from build123d import *

# Parameters (mm, degrees)
SKETCH_1_W               = 164.2
SKETCH_1_H               = 104.2
EXTRUDE_1_DEPTH          = 8
SKETCH_2_R               = 0.3
CUT_EXTRUDE_1_DEPTH      = 98.564440243
CUT_EXTRUDE_2_DEPTH      = 5.9
SKETCH_5_W               = 148.4
SKETCH_5_H               = 100.2
CUT_EXTRUDE_5_DEPTH      = 1.2
SKETCH_6_W               = 164.2
SKETCH_6_H               = 104.2
SKETCH_6_W_2             = 148.4
SKETCH_6_H_2             = 100.2
EXTRUDE_2_DEPTH          = 3
CUT_EXTRUDE_6_DEPTH      = 132.336400133
CUT_EXTRUDE_6_DEPTH_BACK = 132.336400133
SKETCH_7_R               = 0.75
CUT_EXTRUDE_START        = -2
SKETCH_7_3_R             = 1
SKETCH_7_3_R_2           = 0.75
CUT_EXTRUDE_7_DEPTH      = 1
CUT_EXTRUDE_START_2      = 101.2
SKETCH_7_4_R             = 1
SKETCH_7_4_R_2           = 0.75
CUT_EXTRUDE_8_DEPTH      = 1
SKETCH_8_R               = 0.75
CUT_EXTRUDE_9_DEPTH      = 171.644953046
CUT_EXTRUDE_START_3      = -0.9
SKETCH_8_3_R             = 1
SKETCH_8_3_R_2           = 0.75
CUT_EXTRUDE_10_DEPTH     = 1
SKETCH_3_W               = 145.9
SKETCH_3_H               = 96.2
SKETCH_3_W_2             = 10.3
SKETCH_3_H_2             = 30.95
CUT_EXTRUDE_11_DEPTH     = 4.8
SKETCH_9_W               = 164.2
SKETCH_9_H               = 104.2
CUT_EXTRUDE_12_DEPTH     = 2.4


with BuildPart() as part:
    # 草图1 → 凸台-拉伸1 (new body)
    with BuildSketch(Plane(origin=(0, 0, 0), x_dir=(1, 0, 0), z_dir=(0, 1, 0))):
        Rectangle(SKETCH_1_W, SKETCH_1_H)
    extrude(amount=EXTRUDE_1_DEPTH)

    # 草图2 → 切除-拉伸1 (cut, through all)
    with BuildSketch(Plane(origin=(0, 8, 0), x_dir=(1, 0, 0), z_dir=(0, 1, 0))):
        with Locations(Location((-74, 11.5, 0), (0, 0, 270))):
            Circle(SKETCH_2_R)
        with Locations(Location((-74, -11.5, 0), (0, 0, 270))):
            Circle(SKETCH_2_R)
        with BuildLine():
            Line((-76.2, -8.05), (-76.2, 8.05))
            ThreePointArc((-76.2, 8.05), (-74, 10.25), (-71.8, 8.05))
            Line((-71.8, 8.05), (-71.8, -8.05))
            ThreePointArc((-71.8, -8.05), (-74, -10.25), (-76.2, -8.05))
        make_face()
    extrude(amount=-CUT_EXTRUDE_1_DEPTH, mode=Mode.SUBTRACT)

    # 草图2<3> → 切除-拉伸2 (cut)
    with BuildSketch(Plane(origin=(0, 8, 0), x_dir=(1, 0, 0), z_dir=(0, 1, 0))):
        with BuildLine():
            Line((-71.8, 10.95), (-71.8, -10.95))
            ThreePointArc((-71.8, -10.95), (-74, -13.15), (-76.2, -10.95))
            Line((-76.2, -10.95), (-76.2, 10.95))
            ThreePointArc((-76.2, 10.95), (-74, 13.15), (-71.8, 10.95))
        make_face()
    extrude(amount=-CUT_EXTRUDE_2_DEPTH, mode=Mode.SUBTRACT)

    # 草图5 → 切除-拉伸5 (cut)
    with BuildSketch(Plane.XZ):
        with Locations((6, 0)):
            Rectangle(SKETCH_5_W, SKETCH_5_H)
    extrude(amount=-CUT_EXTRUDE_5_DEPTH, mode=Mode.SUBTRACT)

    # 草图6 → 凸台-拉伸2 (add)
    with BuildSketch(Plane.XZ):
        Rectangle(SKETCH_6_W, SKETCH_6_H)
        with BuildLine():
            ThreePointArc((-71.8, -10.95), (-74.1, -13.25), (-76.4, -10.95))
            Line((-76.4, -10.95), (-76.4, -5.229910312))
            ThreePointArc((-76.4, -5.229910312), (-77.793738469, -4.481131324), (-78.35, -3))
            Line((-78.35, -3), (-78.35, 3))
            ThreePointArc((-78.35, 3), (-77.793738469, 4.481131324), (-76.4, 5.229910312))
            Line((-76.4, 5.229910312), (-76.4, 10.95))
            ThreePointArc((-76.4, 10.95), (-74.1, 13.25), (-71.8, 10.95))
            Line((-71.8, 10.95), (-71.8, 8.05))
            Line((-71.8, 8.05), (-71.8, 2.229910312))
            ThreePointArc((-71.8, 2.229910312), (-70.406261531, 1.481131324), (-69.85, 0))
            ThreePointArc((-69.85, 0), (-70.406261531, -1.481131324), (-71.8, -2.229910312))
            Line((-71.8, -2.229910312), (-71.8, -8.05))
            Line((-71.8, -8.05), (-71.8, -10.95))
        make_face(mode=Mode.SUBTRACT)
        with Locations((6, 0)):
            Rectangle(SKETCH_6_W_2, SKETCH_6_H_2, mode=Mode.SUBTRACT)
    extrude(amount=EXTRUDE_2_DEPTH)

    # 草图7 → 切除-拉伸6 (cut, two sides: drawn at the far end of the back side and taken through both)
    with BuildSketch(Plane.XY.offset(-50.1).offset(-CUT_EXTRUDE_6_DEPTH_BACK)):
        with Locations((6, -1)):
            Circle(SKETCH_7_R)
        with Locations((-54, -1)):
            Circle(SKETCH_7_R)
        with Locations((66, -1)):
            Circle(SKETCH_7_R)
    extrude(amount=CUT_EXTRUDE_6_DEPTH + CUT_EXTRUDE_6_DEPTH_BACK, mode=Mode.SUBTRACT)

    # 草图7<3> → 切除-拉伸7 (cut)
    # profile 1 of 3: a face of its own
    with BuildSketch(Plane.XY.offset(-50.1).offset(CUT_EXTRUDE_START)):
        with Locations((6, -1)):
            Circle(SKETCH_7_3_R)
        with Locations((6, -1)):
            Circle(SKETCH_7_3_R_2, mode=Mode.SUBTRACT)
    # profile 2 of 3: a face of its own
    with BuildSketch(Plane.XY.offset(-50.1).offset(CUT_EXTRUDE_START)):
        with Locations((66, -1)):
            Circle(SKETCH_7_3_R)
        with Locations((66, -1)):
            Circle(SKETCH_7_3_R_2, mode=Mode.SUBTRACT)
    # profile 3 of 3: a face of its own
    with BuildSketch(Plane.XY.offset(-50.1).offset(CUT_EXTRUDE_START)):
        with Locations((-54, -1)):
            Circle(SKETCH_7_3_R)
        with Locations((-54, -1)):
            Circle(SKETCH_7_3_R_2, mode=Mode.SUBTRACT)
    extrude(amount=CUT_EXTRUDE_7_DEPTH, mode=Mode.SUBTRACT)

    # 草图7<4> → 切除-拉伸8 (cut)
    # profile 1 of 3: a face of its own
    with BuildSketch(Plane.XY.offset(-50.1).offset(CUT_EXTRUDE_START_2)):
        with Locations((6, -1)):
            Circle(SKETCH_7_4_R)
        with Locations((6, -1)):
            Circle(SKETCH_7_4_R_2, mode=Mode.SUBTRACT)
    # profile 2 of 3: a face of its own
    with BuildSketch(Plane.XY.offset(-50.1).offset(CUT_EXTRUDE_START_2)):
        with Locations((66, -1)):
            Circle(SKETCH_7_4_R)
        with Locations((66, -1)):
            Circle(SKETCH_7_4_R_2, mode=Mode.SUBTRACT)
    # profile 3 of 3: a face of its own
    with BuildSketch(Plane.XY.offset(-50.1).offset(CUT_EXTRUDE_START_2)):
        with Locations((-54, -1)):
            Circle(SKETCH_7_4_R)
        with Locations((-54, -1)):
            Circle(SKETCH_7_4_R_2, mode=Mode.SUBTRACT)
    extrude(amount=CUT_EXTRUDE_8_DEPTH, mode=Mode.SUBTRACT)

    # 草图8 → 切除-拉伸9 (cut, through all)
    with BuildSketch(Plane.ZY.offset(-80.2)):
        with Locations((-35, -1)):
            Circle(SKETCH_8_R)
        with Locations((0, -1)):
            Circle(SKETCH_8_R)
        with Locations((35, -1)):
            Circle(SKETCH_8_R)
    extrude(amount=-CUT_EXTRUDE_9_DEPTH, mode=Mode.SUBTRACT)

    # 草图8<3> → 切除-拉伸10 (cut)
    # profile 1 of 3: a face of its own
    with BuildSketch(Plane.ZY.offset(-80.2).offset(CUT_EXTRUDE_START_3)):
        with Locations((0, -1)):
            Circle(SKETCH_8_3_R)
        with Locations((0, -1)):
            Circle(SKETCH_8_3_R_2, mode=Mode.SUBTRACT)
    # profile 2 of 3: a face of its own
    with BuildSketch(Plane.ZY.offset(-80.2).offset(CUT_EXTRUDE_START_3)):
        with Locations((-35, -1)):
            Circle(SKETCH_8_3_R)
        with Locations((-35, -1)):
            Circle(SKETCH_8_3_R_2, mode=Mode.SUBTRACT)
    # profile 3 of 3: a face of its own
    with BuildSketch(Plane.ZY.offset(-80.2).offset(CUT_EXTRUDE_START_3)):
        with Locations((35, -1)):
            Circle(SKETCH_8_3_R)
        with Locations((35, -1)):
            Circle(SKETCH_8_3_R_2, mode=Mode.SUBTRACT)
    extrude(amount=-CUT_EXTRUDE_10_DEPTH, mode=Mode.SUBTRACT)

    # 草图3 → 切除-拉伸11 (cut)
    with BuildSketch(Plane(origin=(0, 8, 0), x_dir=(1, 0, 0), z_dir=(0, 1, 0))):
        with Locations((5.15, 0)):
            Rectangle(SKETCH_3_W, SKETCH_3_H)
        with Locations((-72.95, 32.625)):
            Rectangle(SKETCH_3_W_2, SKETCH_3_H_2)
        with Locations((-72.95, -32.625)):
            Rectangle(SKETCH_3_W_2, SKETCH_3_H_2)
    extrude(amount=-CUT_EXTRUDE_11_DEPTH, mode=Mode.SUBTRACT)

    # 草图9 → 切除-拉伸12 (cut)
    with BuildSketch(Plane(origin=(0, 8, 0), x_dir=(1, 0, 0), z_dir=(0, 1, 0))):
        Rectangle(SKETCH_9_W, SKETCH_9_H)
    extrude(amount=-CUT_EXTRUDE_12_DEPTH, mode=Mode.SUBTRACT)


solid = part.part
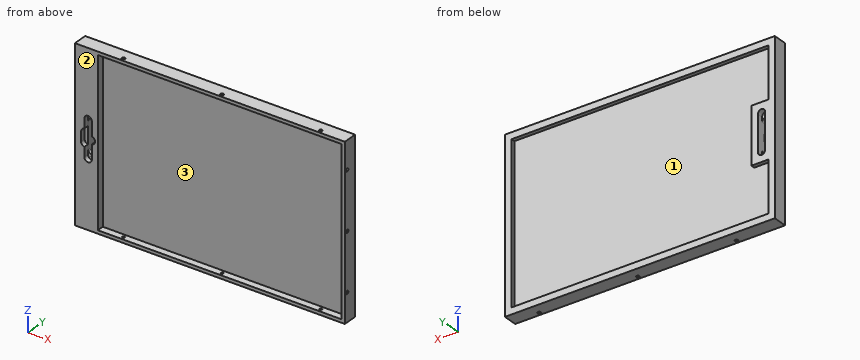
The listing builds one solid part. Answer for the finished solid, in the listing's coordinates (mm). Face numbers are marked on the shaded views. Coordinates: 2 decimals unless noted, no trailing zeros. Loops run counter-clockwise (first coordinate to the right, second up) from the corner with the lowest first, then second, coordinate; pieces in that order, holes last. Notation, with made-up numbers: (22, 43) -> (26, 43) arc R10 ccw to (26, 48) -> close; hole circle Ø9 at (8.25, 77.5). An arc over 180 degrees is marked (long way). Write item = value, one per line. Start each with the question number.
1) A cutting plane is placed at B-B (x = -51). Give the vertices of the cut face in (y, z).
2) Given pin 1 Ø0.9 at (x, y) = (6, -1) entering from +Z; pin 2 Ø2 at (x, z) = (-74.5, 10) entering from +Y; pin 3 Ø1.4 at (y, z) = (-1, 0) entering from +X; pin 4 Ø2 at (x, z) = (-11, -20) entering from -Y, each flat-ended and moving along its own axis, determine where each tip first touches the part or whether it passes through.
3) The mould has two halves that part along Z. Classify the marked faces 1, 2 and 3: released by +Z, released by -Z, zero draft, split by the parting line, or undercut.
4) Straight lines are drawn through the part: line 1 (X direction, y = 3.25, z = 9); line 2 (X direction, y = -1, z = -50.65); line 3 (X direction, y = 0.7, z = -11.5). For each, find the intervals that lie inside material, in ascending order. Write a range as from..to.
5) A cutting plane is placed at A-A (z = 27). Give the vertices of the cut face in (x, y), then the cut area to 3 significant figures.
Responses:
q1.outline = (-3, -52.1) -> (5.6, -52.1) -> (5.6, -48.1) -> (3.2, -48.1) -> (3.2, 48.1) -> (5.6, 48.1) -> (5.6, 52.1) -> (-3, 52.1) -> (-3, 50.1) -> (1.2, 50.1) -> (1.2, -50.1) -> (-3, -50.1) -> close
q2.pin_1 = through
q2.pin_2 = 2.1
q2.pin_3 = -68.2
q2.pin_4 = 1.2
q3.face_1 = undercut
q3.face_2 = zero draft
q3.face_3 = undercut
q4.line_1 = -82.1..-76.2, -71.8..-67.8, 78.1..82.1
q4.line_2 = -82.1..-54.75, -53.25..5.25, 6.75..65.25, 66.75..82.1
q4.line_3 = -82.1..-74.3, -73.7..-68.2, 80.2..82.1
q5.outline = (-82.1, -3) -> (-68.2, -3) -> (-68.2, 1.2) -> (80.2, 1.2) -> (80.2, -3) -> (82.1, -3) -> (82.1, 5.6) -> (78.1, 5.6) -> (78.1, 3.2) -> (-78.1, 3.2) -> (-78.1, 5.6) -> (-82.1, 5.6) -> close
q5.area = 414 mm²
